from build123d import *

# Parameters (mm, degrees)
BOSS_EXTRUDE1_DEPTH = 3
BOSS_EXTRUDE5_DEPTH = 35
BOSS_EXTRUDE6_DEPTH = 3
SKETCH8_W           = 80.8
SKETCH8_H           = 69.3
BOSS_EXTRUDE8_DEPTH = 2
BOSS_EXTRUDE9_DEPTH = 80.8
SKETCH10_W          = 4.5
SKETCH10_H          = 6
CUT_EXTRUDE1_DEPTH  = 5
SKETCH13_W          = 9.8
SKETCH13_H          = 3
CUT_EXTRUDE2_DEPTH  = 5


with BuildPart() as part:
    # Sketch1 → Boss-Extrude1 (new body)
    with BuildSketch(Plane.XY):
        Polygon((30.4, -26.4), (40.4, -26.4), (40.4, 41.4), (-40.4, 41.4), (-40.4, -26.4), (-30.4, -26.4), (-30.4, 31.4), (30.4, 31.4), align=None)
    extrude(amount=-BOSS_EXTRUDE1_DEPTH)

    # Sketch5 → Boss-Extrude5 (add)
    with BuildSketch(Plane.XY):
        Polygon((-40.4, 41.4), (-5, -21.9), (0, -21.9), (5, -21.9), (40.4, 41.4), (40.4, -27.9), (-40.4, -27.9), align=None)
    extrude(amount=-BOSS_EXTRUDE5_DEPTH)

    # Sketch6 → Boss-Extrude6 (add)
    with BuildSketch(Plane.XY):
        Polygon((-40.4, 41.4), (40.4, 41.4), (40.4, -27.9), (30.4, -27.9), (30.4, 31.4), (-30.4, 31.4), (-30.4, -27.9), (-40.4, -27.9), align=None)
    extrude(amount=BOSS_EXTRUDE6_DEPTH)

    # Sketch8 → Boss-Extrude8 (add)
    with BuildSketch(Plane(origin=(0, 0, -35), x_dir=(-1, 0, 0), z_dir=(0, 0, -1))):
        with Locations((0, 6.75)):
            Rectangle(SKETCH8_W, SKETCH8_H)
    extrude(amount=-BOSS_EXTRUDE8_DEPTH)

    # Sketch9 → Boss-Extrude9 (add)
    with BuildSketch(Plane(origin=(40.4, 0, 0), x_dir=(0, 0, -1), z_dir=(1, 0, 0))):
        Polygon((33, -21.9), (33, 41.4), (5, -21.9), align=None)
    extrude(amount=-BOSS_EXTRUDE9_DEPTH)

    # Sketch10 → Cut-Extrude1 (cut)
    with BuildSketch(Plane.XY):
        with Locations((7.05, -24.9)):
            Rectangle(SKETCH10_W, SKETCH10_H)
        with Locations((-7.05, -24.9)):
            Rectangle(SKETCH10_W, SKETCH10_H)
    extrude(amount=-CUT_EXTRUDE1_DEPTH, mode=Mode.SUBTRACT)

    # Sketch13 → Cut-Extrude2 (cut)
    with BuildSketch(Plane.XY.offset(-5)):
        with Locations((-0.1, -23.4)):
            Rectangle(SKETCH13_W, SKETCH13_H)
    extrude(amount=CUT_EXTRUDE2_DEPTH, mode=Mode.SUBTRACT)


solid = part.part
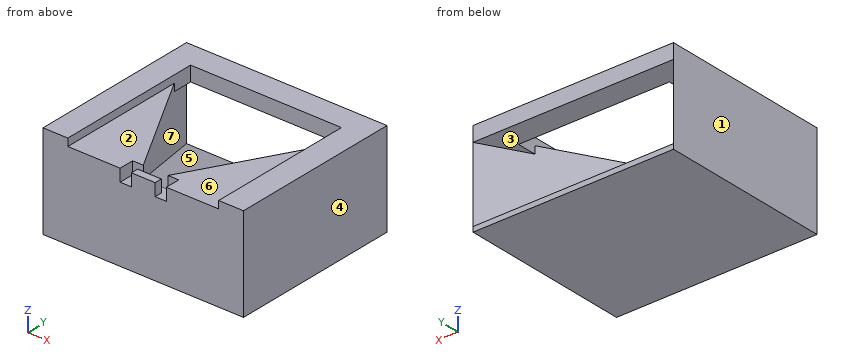
Design review of the part built by this model. Coordinates are the model's own, in mm. Face numbers are marked on the shaded views. A direction names the side the tool comes from. Give positions to 0.01 mm unless a question says otherwise; leave off trailing zeros. Write each loop counter-clockwise with the first axis right and the second up, starting at its lowest first coordinate (ties: lowest second). Pieces come first, ordered by that corner, then holes. Notation, with made-up numbers: M 1.5,-36.75 L 30.5,-36.75 A16 cw 30.5,-5.75 Z; hole C 51.5,78 d9. An arc over 180 degrees is marked long. Answer as a JSON object with one key per item and string values. Group by question number.
1) Clearance check with flat-ended pins moving along their axes: pin 1 Ø7.5 at (x, y) = (-19.5, -6.5) entering from +Z; pin 2 Ø2 at (x, z) = (-7.5, -2.5) entering from -Y. State where each tip first meets the part, or that it passes through.
2) We need section D-D (y = 24.5). Give the boundary of the cut face in (x, z).
3) Tool access review of the marked faces 4, 5, 6 and 7: name each direction out of +Z, -Z, +X, -X, +Y, -Y from which nothing blocks a thin tool from reaching the whole face with its end or side.
4) We need section A-A (x = -24). Give the boundary of the cut face in (y, z), and give its area (3 significant figures).
5) We need section B-B (y = 35). Give the boundary of the cut face in (x, z).
6) For line 1 along Z through (x, y) = (-23, 6.5); line 2 along X through (y, z) = (23, -11); line 3 along X through (y, z) = (-18, -1), list the stretches that pass through material, from the lowest coordinate up.
7) We need section C-C (z = -11). Give the boundary of the cut face in (x, y), and give its area (3 significant figures).
8) Mouldability with a two-part tool opening along Z and no side actions: class the marked faces 1, 2 and 3 as released by +Z, released by -Z, zero draft, split by the parting line, or undercut.
Answer key:
{
 "1": {"pin 1": "stops at z = 0", "pin 2": "stops at y = -21.9"},
 "2": {"outline": "M -40.4,-35 L 40.4,-35 L 40.4,3 L 30.4,3 L 30.4,-3 L 30.95,-3 L 30.95,-25.52 L -30.95,-25.52 L -30.95,-3 L -30.4,-3 L -30.4,3 L -40.4,3 Z"},
 "3": {"face 4": "+Z, -Z, +X, +Y, -Y", "face 5": "+Y", "face 6": "+Z, -Y", "face 7": "none"},
 "4": {"outline": "M -27.9,-35 L 41.4,-35 L 41.4,-33 L 12.07,-20.03 L 12.07,0 L -27.9,0 Z; M 31.4,-3 L 41.4,-3 L 41.4,3 L 31.4,3 Z", "area": "1,710 mm²"},
 "5": {"outline": "M -40.4,-35 L 40.4,-35 L 40.4,3 L -40.4,3 Z; hole M -36.82,-30.17 L 36.82,-30.17 L 36.82,-3 L -36.82,-3 Z"},
 "6": {"line 1": "z = -35 to 0", "line 2": "x = -40.4 to -30.11, 30.11 to 40.4", "line 3": "x = -40.4 to -7.18, 7.18 to 40.4"},
 "7": {"outline": "M -40.4,-27.9 L 40.4,-27.9 L 40.4,41.4 L 12.59,-8.34 L -12.59,-8.34 L -40.4,41.4 Z", "area": "2,960 mm²"},
 "8": {"face 1": "zero draft", "face 2": "released by +Z", "face 3": "undercut"}
}
